from build123d import *

# Parameters (mm, degrees)
F0_R     = 62.992
F1_DEPTH = 43.942
F2_R     = 52.959
F3_DEPTH = 43.942
F4_R     = 6.4897
F5_DEPTH = 63.5


with BuildPart() as f1:
    # F0 (on Top) → F1 (new body)
    with BuildSketch(Plane.XY):
        Circle(F0_R)
    extrude(amount=F1_DEPTH)

    # F2 (on face) → F3 (cut)
    with BuildSketch(Plane.XY.offset(43.942)):
        Circle(F2_R)
    extrude(amount=-F3_DEPTH, mode=Mode.SUBTRACT)

    # F4 (on Front) → F5 (cut, symmetric)
    with BuildSketch(Plane.XZ):
        with Locations((0, 43.091593)):
            Circle(F4_R)
    extrude(amount=F5_DEPTH, both=True, mode=Mode.SUBTRACT)


solid = f1.part
The model under review builds one solid part; all positions refer to its coordinate system, in mm. Round coordinates to 2 decimals unless told otherwise and drop trailing zeros. Loops run counter-clockwise (first coordinate to the right, second up) from the corner with the lowest first, then second, coordinate; pieces in that order, holes last. Notation, with made-up numbers: M -36.5,66 L 9.5,66 A28 ccw 9.5,98 Z; hole C 30,-17 d5. An arc over 180 degrees is marked long. Answer as CSV lines item,"result".
1. To check wall thickness, follow L1, parallel to X at y = 0, z = 24; L2, parallel to X at y = 48, z = 15. State the ranges of each line that lie inside material, in increasing order. Write a range as [from, to].
Outcome:
L1,"x = [-62.99, -52.96], [52.96, 62.99]"
L2,"x = [-40.79, -22.38], [22.38, 40.79]"
2. We need section B-B (x = 0). Give the boundary of the cut face in (y, z), plus the area to 3 significant figures.
Outcome:
outline,"M -62.99,0 L -52.96,0 L -52.96,36.6 L -62.99,36.6 Z; M 52.96,0 L 62.99,0 L 62.99,36.6 L 52.96,36.6 Z"
area,"734 mm2"
3. Insertion check: pin 1 Ø2 at (y, z) = (-23.5, 5) entering from +X; pin 2 Ø8 at (x, z) = (-22.5, 17.5) entering from -Y; pin 3 Ø10 at (x, z) = (5, 6) entering from +Y; pin 4 Ø4 at (x, y) = (49, -5) entering from -Z. Each pin has a flat end and moves straight along its axis. Give the tip position at first contact, or say it passes through.
Outcome:
pin 1,"stops at x = 58.84"
pin 2,"stops at y = -60.21"
pin 3,"stops at y = 62.99"
pin 4,"passes through"
4. Draft analysis for pull direction Y (two halves, no side actions). For faces 1 (the face through (50.513, 15.907, 22.279)), 2 (the face through (-13.655, -61.494, 21.663)), 3 (the face through (-54, 0, 43.942)), state which applies: pulls with the +Y half, pulls with the -Y half, needs draft (parallel to the pull), parting line crosses it, or undercut.
Outcome:
face 1,"undercut"
face 2,"parting line crosses it"
face 3,"needs draft"
5. We need section C-C (z = 10.5). Give the boundary of the cut face in (x, y).
Outcome:
outline,"C 0,0 d125.98; hole C 0,0 d105.92"
6. We need section A-A (y = 0). Give the boundary of the cut face in (x, z).
Outcome:
outline,"M -62.99,0 L -52.96,0 L -52.96,43.94 L -62.99,43.94 Z; M 52.96,0 L 62.99,0 L 62.99,43.94 L 52.96,43.94 Z"
